Verification items for the finished model (mm, model axes). Face numbers are marked on the shaded views. Coordinates: 2 decimals unless noted, no trailing zeros. Loops run counter-clockwise (first coordinate to the right, second up) from the corner with the lowest first, then second, coordinate; pieces in that order, holes last. Notation, with made-up numbers: (-5.5, 29.25) -> (38.5, 29.25) arc R23 ccw to (38.5, 44.25) -> close; hole circle Ø1 at (-33.75, -0.75). An arc over 180 degrees is marked (long way). Use CSV: the item, a comma, the result in double quotes. Start each with the question number.
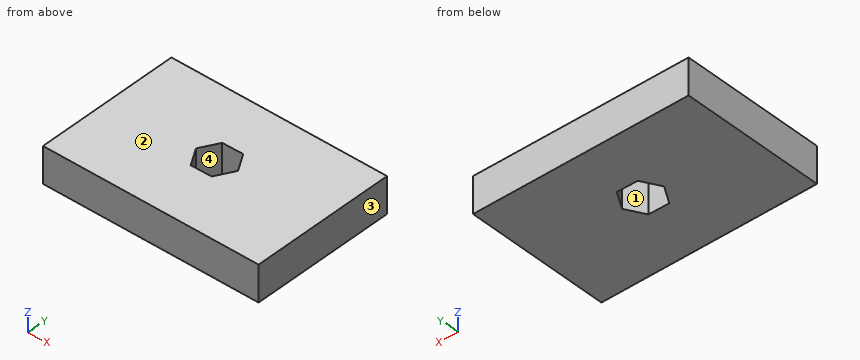
```python
from build123d import *

# Parameters (mm, degrees)
SKETCH1_W           = 76.2
SKETCH1_H           = 50.8
BOSS_EXTRUDE1_DEPTH = 6.35
CUT_EXTRUDE1_DEPTH  = 13.7


with BuildPart() as part:
    # Sketch1 → Boss-Extrude1 (new body, symmetric)
    with BuildSketch(Plane.XY):
        Rectangle(SKETCH1_W, SKETCH1_H)
    extrude(amount=BOSS_EXTRUDE1_DEPTH, both=True)

    # Sketch3 → Cut-Extrude1 (cut, through all)
    with BuildSketch(Plane.XY.offset(6.35)):
        Polygon((-3.5620661, -5.630417032), (3.769306023, -5.510767006), (7.331372123, 0.89821251), (3.5620661, 7.187542), (-3.769306023, 7.067891975), (-7.331372123, 0.658912459), align=None)
    extrude(amount=-CUT_EXTRUDE1_DEPTH, mode=Mode.SUBTRACT)


solid = part.part
```
1. Scan lines: line 1 (Y direction, x = 0, z = 2.75); line 2 (X direction, y = -0.5, z = -4); line 3 (X direction, y = -3, z = 2.25). Record each from-to range of solid material in increasing order.
2. Release check for a two-part mould opening along X. For the marked faces 1, 2, 3 and 4 record: released by +X, released by -X, zero draft, split by the parting line, or undercut.
3. Cross-section at A-A, the plane y = -0.5. Record the boundary of the cut face in (x, z).
4. Cross-section at B-B, the plane z = 2.5. Record the boundary of the cut face in (x, y).
Solution:
1,line 1,"y = -25.4 to -5.57, 7.13 to 25.4"
1,line 2,"x = -38.1 to -6.64, 6.55 to 38.1"
1,line 3,"x = -38.1 to -5.14, 5.16 to 38.1"
2,face 1,"undercut"
2,face 2,"zero draft"
2,face 3,"released by +X"
2,face 4,"undercut"
3,outline,"(-38.1, -6.35) -> (-6.64, -6.35) -> (-6.64, 6.35) -> (-38.1, 6.35) -> close; (6.55, -6.35) -> (38.1, -6.35) -> (38.1, 6.35) -> (6.55, 6.35) -> close"
4,outline,"(-38.1, -25.4) -> (38.1, -25.4) -> (38.1, 25.4) -> (-38.1, 25.4) -> close; hole (-7.33, 0.66) -> (-3.56, -5.63) -> (3.77, -5.51) -> (7.33, 0.9) -> (3.56, 7.19) -> (-3.77, 7.07) -> close"
